Autodesk Fusion 360 part; units mm, degrees
sketch "草图6" plane through (0, 0, 0) normal (0, 0, 1) x (1, 0, 0)
  line L0 (4, 0) -> (12, 0)
  line L1 (16, 4) -> (16, 41)
  line L2 (12, 45) -> (4, 45)
  line L3 (0, 41) -> (0, 4)
  arc A0 (4, 45) -> (0, 41) centre (4, 41) ccw
  arc A1 (16, 41) -> (12, 45) centre (12, 41) ccw
  arc A2 (0, 4) -> (4, 0) centre (4, 4) ccw
  arc A3 (12, 0) -> (16, 4) centre (12, 4) ccw
  line L4 (25, 31.5418) -> (33, 31.5418)
  line L5 (33, 31.5418) -> (33, 16.5418)
  line L6 (33, 16.5418) -> (25, 16.5418)
  line L7 (25, 16.5418) -> (25, 31.5418)
  line L8 (-15, 52.2379) -> (45, 52.2379)
  line L9 (45, 52.2379) -> (45, -7.7621)
  line L10 (45, -7.7621) -> (-15, -7.7621)
  line L11 (-15, -7.7621) -> (-15, 52.2379)
  line L12 (45, -7.7621) -> (-15, 52.2379) construction
  line L13 (-15, -7.7621) -> (45, 52.2379) construction
  circle A4 centre (15, 22.2379) radius 43.1
  point P0 (16, 0)
  point P1 (0, 45)
  dimension "d37" = 4
  dimension "d38" = 4
  dimension "d39" = 4
  dimension "d40" = 4
  dimension "d41" = 45
  dimension "d42" = 16
  dimension "d43" = 8
  dimension "d44" = 15
  dimension "d45" = 60
  dimension "d55" = 60
  dimension "d56" = 86.2
extrude "拉伸5" add sketch "草图6" along normal blind 5 contours L8 L9 L10 L11
sketch "草图7" plane through (0, 45, 0) normal (0, -1, 0) x (1, 0, 0)
  line L0 (4, 0) -> (12, 0)
  line L1 (12, 0) -> (12, 5)
  line L2 (12, 5) -> (4, 5)
  line L3 (4, 5) -> (4, 0)
  circle A0 centre (8, 5) radius 1.6
  dimension "d48" = 3.2
extrude "拉伸6" cut sketch "草图7" along normal blind -10 and the other way blind -55 contours L2 A0 picked at (7.5748, 4.2826)
extrude "拉伸7" add sketch "草图6" along normal blind 5 contours A4
sketch "草图10" plane through (0, 0, 0) normal (0, 0, -1) x (1, 0, 0)
  circle A0 centre (15, -22.2379) radius 43.1
  arc A1 (16, -4) -> (12, 0) centre (12, -4) ccw
  line L0 (16, -4) -> (16, -41)
  arc A2 (12, -45) -> (16, -41) centre (12, -41) ccw
  line L1 (12, -45) -> (4, -45)
  arc A3 (0, -41) -> (4, -45) centre (4, -41) ccw
  line L2 (0, -41) -> (0, -4)
  arc A4 (4, 0) -> (0, -4) centre (4, -4) ccw
  line L3 (4, 0) -> (12, 0)
  line L4 (25, -16.5418) -> (33, -16.5418)
  line L5 (33, -16.5418) -> (33, -31.5418)
  line L6 (33, -31.5418) -> (25, -31.5418)
  line L7 (25, -31.5418) -> (25, -16.5418)
  circle A5 centre (15, -22.2379) radius 35
  circle A6 centre (15, -57.2379) radius 3
  circle A7 centre (15, -57.2379) radius 1.35
  circle A8 centre (50, -22.2379) radius 3
  circle A9 centre (50, -22.2379) radius 1.35
  circle A10 centre (15, 12.7621) radius 3
  circle A11 centre (15, 12.7621) radius 1.35
  circle A12 centre (-20, -22.2379) radius 3
  circle A13 centre (-20, -22.2379) radius 1.35
  line L8 (-7.4138, -45.6983) -> (-7.8923, -46.1073)
  line L9 (-6.756, -46.4514) -> (-7.1427, -46.7964)
  arc A14 (-6.756, -46.4514) -> (-7.4138, -45.6983) centre (-7.0889, -46.0783) ccw
  arc A15 (-7.8923, -46.1073) -> (-7.1427, -46.7964) centre (-8.8265, -47.8757) ccw
  arc A16 (38.8694, -45.1301) -> (39.5585, -44.3806) centre (40.6378, -46.0644) ccw
  line L10 (38.4604, -44.6517) -> (38.8694, -45.1301)
  arc A17 (39.2135, -43.9939) -> (38.4604, -44.6517) centre (38.8404, -44.3268) ccw
  line L11 (39.2135, -43.9939) -> (39.5585, -44.3806)
  arc A18 (37.8923, 1.6315) -> (37.1427, 2.3206) centre (38.8265, 3.3999) ccw
  line L12 (37.4138, 1.2225) -> (37.8923, 1.6315)
  arc A19 (36.756, 1.9756) -> (37.4138, 1.2225) centre (37.0889, 1.6025) ccw
  line L13 (36.756, 1.9756) -> (37.1427, 2.3206)
  arc A20 (-8.8694, 0.6544) -> (-9.5585, -0.0951) centre (-10.6378, 1.5886) ccw
  line L14 (-8.4604, 0.1759) -> (-8.8694, 0.6544)
  arc A21 (-9.2135, -0.4818) -> (-8.4604, 0.1759) centre (-8.8404, -0.149) ccw
  line L15 (-9.2135, -0.4818) -> (-9.5585, -0.0951)
  dimension "d59" = 70
  dimension "d60" = 6
  dimension "d61" = 2.7
  dimension "d63" = 360
  dimension "d68" = 4
  dimension "d69" = 1
  dimension "d71" = 360
extrude "拉伸8" cut sketch "草图10" against normal up to surface (5 mm away) contours A5 A9 | A5 A9 | A5 A11 | A5 A11 | A5 A7 | A5 A7 | A5 A13 | A5 A13
extrude "拉伸9" cut sketch "草图10" against normal blind 3 contours A5 A8 A9 | A5 A8 A9 | A5 A10 A11 | A5 A10 A11 | A5 A6 A7 | A5 A6 A7 | A5 A12 A13 | A5 A12 A13
sketch "草图11" plane through (0, 0, 0) normal (0, 0, -1) x (1, 0, 0)
  circle A0 centre (50, -22.2379) radius 3
  circle A1 centre (-20, -22.2379) radius 3
  circle A2 centre (15, -57.2379) radius 3
  circle A3 centre (15, 12.7621) radius 3
  circle A4 centre (15, -22.2379) radius 43.1
  arc A5 (16, -4) -> (12, 0) centre (12, -4) ccw
  line L0 (16, -4) -> (16, -41)
  arc A6 (12, -45) -> (16, -41) centre (12, -41) ccw
  line L1 (12, -45) -> (4, -45)
  arc A7 (0, -41) -> (4, -45) centre (4, -41) ccw
  line L2 (0, -41) -> (0, -4)
  arc A8 (4, 0) -> (0, -4) centre (4, -4) ccw
  line L3 (4, 0) -> (12, 0)
  line L4 (25, -16.5418) -> (33, -16.5418)
  line L5 (33, -16.5418) -> (33, -31.5418)
  line L6 (33, -31.5418) -> (25, -31.5418)
  line L7 (25, -31.5418) -> (25, -16.5418)
  circle A9 centre (15, -22.2379) radius 35
  circle A10 centre (39.6014, 2.6573) radius 1.3
  circle A11 centre (-9.8952, 2.3635) radius 1.3
  circle A12 centre (-9.6014, -47.1331) radius 1.3
  circle A13 centre (39.8952, -46.8393) radius 1.3
  dimension "d74" = 2.6
  dimension "d76" = 360
extrude "拉伸11" cut sketch "草图11" against normal blind 5 contours A9 A10 | A9 A10 | A9 A13 | A9 A13 | A9 A11 | A9 A11 | A9 A12 | A9 A12
The listing builds one solid part. Answer for the finished solid, in the listing's coordinates (mm). A direction names the side the tool comes from. Give positions to 0.01 mm unless a question says otherwise; leave off trailing zeros. Write each loop counter-clockwise with the first axis right and the second up, starting at its lowest first coordinate (ties: lowest second). Pieces come first, ordered by that corner, then holes.
Item 1: Which of the six approach directions +Z, -Z, +X, -X, +Y, -Y give full straight-line access (tool end or side, diameter ignored) to faces 1 (the cylindrical face through (1.141, 43.797, 2.465)), 2 (the cylindrical face through (8, 48.6, 3.4)), 3 (the flat face through (-19, 24, 3))?
Item 2: Find the intervals of material crossed by line 1 along Y through (x, z) = (15, 3.55); line 2 along X through (y, z) = (47, 1.55); line 3 along Y through (x, z) = (15, 1.1), in increasing order.
Item 3: Determine the mould class of faces 4 (the cylindrical face through (5.657, 64.313, 2.465)), 5 (the flat face through (24, 23, 5)), 6 (the flat face through (8, 0, 2)), 7 (the cylindrical face through (47.003, 22.106, 1.479)) for opening direction X: released by +X, released by -X, zero draft, split by the parting line, or undercut.
Item 4: Section D-D, the plane z = 1.2 is taken. Count the separate pieces of the cut face and the enclosed holes in it, plus the area to 3 significant figures.
Item 5: Section C-C, the plane x = 15 is taken. Write down the section's boundary in (y, z), plus the area to 3 significant figures.
Item 6: Section B-B, the plane x = 50 is taken. Write down the section's boundary in (y, z), plus the area to 3 significant figures.
Item 7: Section A-A, the plane y = 27.5 is taken. Write down the section's boundary in (x, z).
Item 8: Flat-ended cylindrical pins translate along their axes: P1, Ø2.5, axis at x = 39.9, y = 46.84, coming from the +Z side; P2, Ø1, axis at x = 16, z = 2, coming from the -Y side; P3, Ø1.5, axis at x = 9.5, z = 2.5, coming from the -Y side; P4, Ø1.8, axis at x = 7.5, z = 4.5, coming from the -Y side. Find the tip coordinate at first contact, or state that the pin passes through.
Completed:
1. face 1: +Z, -Z
1. face 2: +Z
1. face 3: -Z
2. line 1: y = -20.86 to -14.11, -11.41 to 1.35, 43.65 to 55.89, 58.59 to 65.34
2. line 2: x = -20.28 to -10.89, -8.31 to 38.61, 41.19 to 50.28
2. line 3: y = -20.86 to -15.76, -9.76 to 1.35, 43.65 to 54.24, 60.24 to 65.34
3. face 4: split by the parting line
3. face 5: zero draft
3. face 6: undercut
3. face 7: undercut
4. separate pieces: 1
4. enclosed holes: 10
4. area: 4,880 mm2
5. outline: (-20.86, 0) - (-15.76, 0) - (-15.76, 3) - (-14.11, 3) - (-14.11, 5) - (-20.86, 5) - close; (-11.41, 3) - (-9.76, 3) - (-9.76, 0) - (1.35, 0) - (1.35, 5) - (-11.41, 5) - close; (43.65, 0) - (54.24, 0) - (54.24, 3) - (55.89, 3) - (55.89, 5) - (43.65, 5) - close; (58.59, 3) - (60.24, 3) - (60.24, 0) - (65.34, 0) - (65.34, 5) - (58.59, 5) - close
5. area: 173 mm2
6. outline: (-2.91, 0) - (19.24, 0) - (19.24, 3) - (20.89, 3) - (20.89, 5) - (-2.91, 5) - close; (23.59, 3) - (25.24, 3) - (25.24, 0) - (47.39, 0) - (47.39, 5) - (23.59, 5) - close
6. area: 228 mm2
7. outline: (-27.78, 0) - (0, 0) - (0, 5) - (-27.78, 5) - close; (16, 0) - (25, 0) - (25, 5) - (16, 5) - close; (33, 0) - (57.78, 0) - (57.78, 5) - (33, 5) - close
8. P1: passes through
8. P2: stops at y = -20.86
8. P3: stops at y = -20.6
8. P4: stops at y = -20.35
